Geometry check sheet. Reference: the model listing, model coordinates, mm. Face numbers are marked on the shaded views. A direction names the side the tool comes from. Coordinates: 2 decimals unless noted, no trailing zeros. Loops run counter-clockwise (first coordinate to the right, second up) from the corner with the lowest first, then second, coordinate; pieces in that order, holes last. Notation, with made-up numbers: (20, 68.5) - (65, 68.5) arc R18 ccw to (65, 101.5) - close; hole circle Ø1 at (12.5, 49). An arc over 180 degrees is marked (long way). One line per item, written item: value.
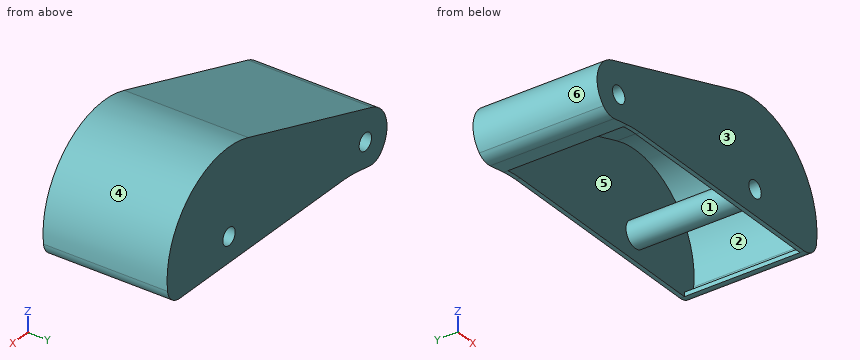
from build123d import *

# Parameters (mm, degrees)
F0_R        = 5
F1_DEPTH    = 73
F2_T1_DEPTH = 73
F3_R        = 10
F4_T        = 2.5


# Not quite as in the source:
# - a fillet or chamfer that OpenCascade refuses, or shapes differently, is made with other operations: its cross-section is extruded or revolved along the edge and cut away or added
# - a shell that OpenCascade refuses in one call is made with other operations: the cavity is built on its own and cut out


with BuildPart() as f1:
    # F0 (on Front) → F1 (new body)
    with BuildSketch(Plane.XZ):
        with BuildLine():
            Line((105.4664104798, -2.1604888337), (110.723299262, -2.1771916507))
            ThreePointArc((110.723299262, -2.1771916507), (98.0443002081, 48.2472921113), (47.4300209604, 60.1460448152))
            Line((47.4300209604, 60.1460448152), (-52.5831548864, 27.4585928761))
            ThreePointArc((-52.5831548864, 27.4585928761), (-64.6091493054, 11.9687796957), (-54.7073812284, -4.9579401011))
            Line((-54.7073812284, -4.9579401011), (-34.93893119, -1.7143761565))
            Line((-34.93893119, -1.7143761565), (20.3665836392, -1.8900994658))
            ThreePointArc((20.3665836392, -1.8900994658), (55.6091219512, 57.015037844), (107.9630298197, 12.6199926356))
            ThreePointArc((107.9630298197, 12.6199926356), (107.3344853384, 5.1250653412), (105.4664104798, -2.1604888337))
        make_face()
        with Locations((-47.1466017857, 10.8244746133)):
            Circle(F0_R, mode=Mode.SUBTRACT)
        with BuildLine():
            Line((20.3665836392, -1.8900994658), (105.4664104798, -2.1604888337))
            ThreePointArc((105.4664104798, -2.1604888337), (107.3344853384, 5.1250653412), (107.9630298197, 12.6199926356))
            ThreePointArc((107.9630298197, 12.6199926356), (55.6091219512, 57.015037844), (20.3665836392, -1.8900994658))
        make_face()
        with Locations((62.9630298197, 12.6199926356)):
            Circle(F0_R, mode=Mode.SUBTRACT)
    extrude(amount=F1_DEPTH)

    # F2: fillet of radius 60 on 1 edges, made by hand

    # F2_s2 → F2_t1 (join)
    with BuildSketch(Plane.XZ):
        with BuildLine():
            add(Edge.make_bspline(
                [(-39.8587548674, -2.52161004), (-34.93893119, -1.7143761565), (-29.9533479112, -1.7302169492)],
                knots=[0, 0, 0, 1, 1, 1], degree=2, weights=[1, 1, 1]))
            Line((-29.9533479112, -1.7302169492), (-34.93893119, -1.7143761565))
            Line((-34.93893119, -1.7143761565), (-39.8587548674, -2.52161004))
        make_face()
    extrude(amount=F2_T1_DEPTH)

    # F3
    f3_edges = [f1.edges().sort_by_distance(p)[0] for p in [
        (110.723299, -36.5, -2.177192),
        (-54.707381, -36.5, -4.95794),
    ]]
    fillet(f3_edges, radius=F3_R)

    # F4: shell of thickness 2.5, made by hand


with BuildPart() as f4_core1:
    # F4_t2: copy of F1
    add(f1.part)

    # the walls: a layer under each face that stays
    f4_faces = [f4_core1.faces().sort_by_distance(p)[0] for p in [
        (94.683390136, -36.5, 51.2699440121),
        (24.158214017, 0, 29.0813282585),
        (109.3014464934, -36.5, 0.3569505301),
        (-2.576566963, -36.5, 43.8023188457),
        (24.158214017, -73, 29.0813282585),
        (-64.1583335829, -36.5, 14.9294692855),
        (-55.554318165, -36.5, -3.9702240205),
        (-45.3554663929, -36.5, -3.4234984168),
        (-52.1466017857, -36.5, 10.8244746133),
        (57.9630298197, -36.5, 12.6199926356),
    ]]
    thicken(f4_faces, amount=-F4_T, mode=Mode.SUBTRACT)


with BuildPart() as f1_1:
    add(f1.part)

    # what is left inside the walls is the cavity
    f4_cavity = [f4_core1.part.solids().sort_by_distance(p)[0] for p in [
        (36.346225, -47.833333, -1.915872),
    ]]
    add(f4_cavity, mode=Mode.SUBTRACT)


solid = f1_1.part
(1) Material ranges on probe 1 along Y at (x, z) = (8, 4); probe 2 along Z at (x, y) = (67, -26); probe 3 along X at (y, z) = (-21, 7), recorded low to high. Write a range as from..to.
Reply:
probe 1: -73..-70.5, -2.5..0
probe 2: 6.3..9.67, 15.57..18.94, 59.95..62.46
probe 3: -64.22..-61.65, -53.6..-50.37, -43.93..-40.69, 58..67.93, 110.13..112.65
(2) Go/stop test with flat-tipped pins: pin 1 Ø2 at (x, y) = (-26.5, -55.5) entering from +Z; pin 2 Ø10 at (x, y) = (-40, -16) entering from -Z; pin 3 Ø12 at (x, y) = (48, -46) entering from +Z. Record where each tip stops, or that it passes through.
Reply:
pin 1: z = 36.31
pin 2: z = -3.37
pin 3: z = 61.81
(3) Cross-section at C-C on x = 9. Record the cut outline in (y, z), and give its area (3 significant figures).
Reply:
outline: (-73, -1.85) - (-70.5, -1.85) - (-70.5, 44.96) - (-2.5, 44.96) - (-2.5, -1.85) - (0, -1.85) - (0, 47.59) - (-73, 47.59) - close
area: 426 mm2
(4) Access from +Z, -Z, +X, -X, +Y, -Y to the whole of each face (thin tool, end or side, straight path). Record for the marked faces 5 and 6.
Reply:
face 5: none
face 6: -X, +Y, -Y
(5) Cross-section at B-B on z = 49.5. Record the cut outline in (x, y).
Reply:
outline: (14.86, -73) - (96.72, -73) - (96.72, 0) - (14.86, 0) - close; hole (22.9, -70.5) - (92.9, -70.5) - (92.9, -2.5) - (22.9, -2.5) - close
(6) Release check for a two-part mould opening along X. For the marked faces 1, 2, 3 and 4 record: pulls with the +X half, pulls with the -X half, needs draft (parallel to the pull), parting line crosses it, or undercut.
Reply:
face 1: undercut
face 2: undercut
face 3: needs draft
face 4: parting line crosses it
(7) Cross-section at D-D on z = 32.5. Record the cut outline in (x, y).
Reply:
outline: (-37.16, -73) - (108.84, -73) - (108.84, 0) - (-37.16, 0) - close; hole (-29.11, -70.5) - (106.1, -70.5) - (106.1, -2.5) - (-29.11, -2.5) - close
(8) Cross-section at A-A on y = -45. Record the cut outline in (x, z), and give its area (3 significant figures).
Reply:
outline: (-59.57, -1.5) arc R10 ccw to (-50.85, -4.33) - (-39.86, -2.52) - (-40.26, -0.05) - (-51.26, -1.86) arc R7.5 cw to (-57.8, 0.26) arc R15 cw to (-51.81, 25.08) - (48.21, 57.77) arc R47.5 cw to (110.12, 6.95) arc R7.5 cw to (102.65, 0.35) - (102.65, -2.15) arc R10 ccw to (112.61, 6.66) arc R50 ccw to (47.43, 60.15) - (-52.58, 27.46) arc R17.5 ccw to start; circle Ø15 at (-47.15, 10.82); circle Ø15 at (62.96, 12.62); hole circle Ø10 at (-47.15, 10.82); hole circle Ø10 at (62.96, 12.62)
area: 867 mm2
